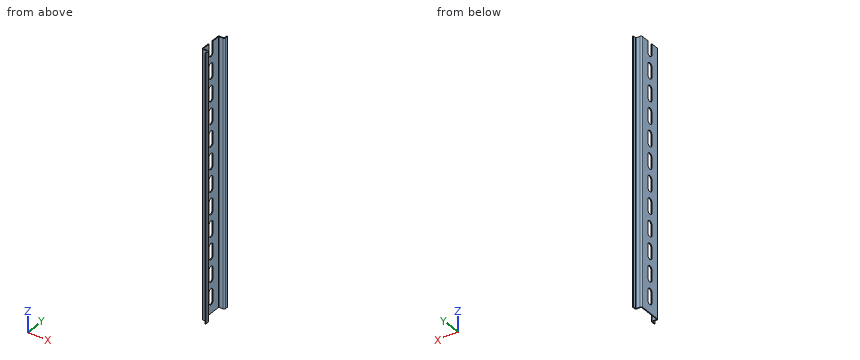
Autodesk Inventor part; units mm, degrees
ref_plane "YZ Plane" through (0, 0, 0) normal (1, 0, 0) x (0, 1, 0)
ref_plane "XZ Plane" through (0, 0, 0) normal (0, 1, 0) x (-1, 0, 0)
ref_plane "XY Plane" through (0, 0, 0) normal (0, 0, 1) x (1, 0, 0)
sketch "Sketch2" plane through (0, 0, 0) normal (0, 0, 1) x (1, 0, 0)
  line L0 (3.5814, 15.9041) -> (4.5814, 15.9041)
  line L1 (4.5814, 15.9041) -> (4.5814, 10.9041)
  line L2 (4.5814, 10.9041) -> (-1.9186, 10.9041)
  line L3 (-1.9186, 10.9041) -> (-1.9186, -14.0959)
  line L4 (-1.9186, -14.0959) -> (4.5814, -14.0959)
  line L5 (4.5814, -14.0959) -> (4.5814, -19.0959)
  line L6 (4.5814, -19.0959) -> (3.5814, -19.0959)
  line L7 (3.5814, -19.0959) -> (3.5814, -15.0959)
  line L8 (3.5814, -15.0959) -> (-2.9186, -15.0959)
  line L9 (-2.9186, -15.0959) -> (-2.9186, 11.9041)
  line L10 (-2.9186, 11.9041) -> (3.5814, 11.9041)
  line L11 (3.5814, 11.9041) -> (3.5814, 15.9041)
  dimension "d0" = 1
  dimension "d1" = 35
  dimension "d2" = 27
  dimension "d3" = 1
  dimension "d4" = 1
  dimension "d5" = 1
  dimension "d6" = 1
  dimension "d7" = 4
  dimension "d8" = 7.5
extrude "Main" add sketch "Sketch2" along normal blind 300
fillet "Fillet2" radius 1.5875 4 edges at (4.5814, 10.9041, 150) (-2.9186, 11.9041, 150) (4.5814, -14.0959, 150) (-2.9186, -15.0959, 150)
fillet "Fillet3" radius 0.7937 4 edges at (3.5814, -15.0959, 150) (-1.9186, 10.9041, 150) (3.5814, 11.9041, 150) (-1.9186, -14.0959, 150)
sketch "Sketch3" plane through (-1.9186, -13.3022, 0) normal (1, 0, 0) x (0, 0, -1)
  line L0 (0, 23.4125) -> (0, 0)
  line L1 (-12.5, 8.5563) -> (-24.2, 8.5563)
  line L2 (-27.35, 11.7063) -> (-27.35, 11.7062)
  line L3 (-24.2, 14.8562) -> (-12.5, 14.8563)
  line L4 (-9.35, 11.7063) -> (-9.35, 11.7063)
  arc A0 (-24.2, 14.8562) -> (-27.35, 11.7062) centre (-24.2, 11.7062) ccw
  arc A1 (-27.35, 11.7063) -> (-24.2, 8.5563) centre (-24.2, 11.7063) ccw
  arc A2 (-12.5, 8.5563) -> (-9.35, 11.7063) centre (-12.5, 11.7063) ccw
  arc A3 (-9.35, 11.7063) -> (-12.5, 14.8563) centre (-12.5, 11.7063) ccw
  line L5 (0, 29.2063) -> (-300, 29.2063)
  dimension "d14" = 3.15
  dimension "d15" = 6.3
  dimension "d16" = 18
  dimension "d17" = 17.5
  dimension "d18" = 12.5
extrude "Extrusion2" cut sketch "Sketch3" against normal through all
pattern_linear "Rectangular Pattern1" count 30 spacing 25 along (0, 0, 1) of "Extrusion2"
equation "\"d0\" = DINWidth"
equation "\"d1\" = DINHeight"
equation "\"d2\" = DINHeightBack"
equation "\"d3\" = DINWidth"
equation "\"d4\" = DINWidth"
equation "\"d5\" = DINWidth"
equation "\"d6\" = DINWidth"
equation "\"d7\" = -0.5 * d2 + 0.5 * d1"
equation "\"d8\" = DINDepth"
equation "\"d14\" = 0.5 * SlotHeight"
equation "\"d15\" = SlotHeight"
equation "\"d16\" = SlotLength"
equation "\"d17\" = 0.5 * DINHeight"
equation "\"d18\" = 0.5 * SlotSpacing"
equation "\"d23\" = SlotSpacing"
equation "\"DINLength\" = 76.2"
equation "\"DINHeight\" = 35"
equation "\"DINHeightBack\" = 27"
equation "\"DINDepth\" = 7.5"
equation "\"SlotHeight\" = 6.3"
equation "\"SlotLength\" = 18"
equation "\"SlotSpacing\" = 25"
equation "\"DINWidth\" = 1"
properties part number "Din Rail_300" material "Латунь светло-желтая"
Can you work these out from the model? Positions are in its coordinate system, mm. Give positions to 0.01 mm unless a question says otherwise; leave off trailing zeros. Order: outer loops, then holes, each group sorted by start corner. A loop starts at its lowest first (then second) coordinate and runs counter-clockwise, first axis right, second up. Notation, with made-up numbers: (78, -22.5) - (108, -22.5) arc R23 cw to (108, -12.5) - close; hole circle Ø5 at (84.25, 59.5). An arc over 180 degrees is marked (long way). Use a Markdown table: item, result. Add a question column.
Q1. Please list where these lines run through material, in increasing order: line 1 along Y through (x, z) = (0.5, 196.5); line 2 along X through (y, z) = (2, 164.5); line 3 along X through (y, z) = (14, 21).
Q2. If we section it at A-A on x = 1: Write out the boundary of the cut face in (y, z).
Q3. If we section it at B-B on y = -7.5: Write out the boundary of the cut face in (x, z).
Q4. I'm going to push flat-ended pins straight in: pin 1 (1.1 mm diameter, centred on x = -2.5, z = 266.5, fed in from -Y); pin 2 (0.5 mm diameter, centred on x = -2.5, z = 166, fed in from -Y); pin 3 (1 mm diameter, centred on x = 0, z = 74.5, fed in from -Y). Where does each tip first touch, or does it pass through?
Answers follow:
| question | item | result |
|---|---|---|
| 1 | line 1 | y = -15.1 to -14.1, 10.9 to 11.9 |
| 1 | line 2 | x = -2.92 to -1.92 |
| 1 | line 3 | x = 3.58 to 4.58 |
| 2 | outline | (-15.1, 0) - (-14.1, 0) - (-14.1, 300) - (-15.1, 300) - close; (10.9, 0) - (11.9, 0) - (11.9, 300) - (10.9, 300) - close |
| 3 | outline | (-2.92, 0) - (-1.92, 0) - (-1.92, 300) - (-2.92, 300) - close |
| 4 | pin 1 | stops at y = -14.97 |
| 4 | pin 2 | stops at y = -14.8 |
| 4 | pin 3 | stops at y = -15.1 |
